The listing builds one solid part. Answer for the finished solid, in the listing's coordinates (mm). A direction names the side the tool comes from. Give positions to 0.01 mm unless a question says otherwise; leave off trailing zeros. Loops run counter-clockwise (first coordinate to the right, second up) from the corner with the lowest first, then second, coordinate; pieces in that order, holes last. Notation, with made-up numbers: M -35.75,-4.5 L -14.75,-4.5 A17 cw -14.75,11.5 Z; hole C 87,39.5 d8. An arc over 180 degrees is marked long. Return JSON: item names as keys, results as strings.
from build123d import *

# Parameters (mm, degrees)
F0_R     = 6.25
F0_R_2   = 2.5
F1_DEPTH = 14
F2_W     = 3.733449
F2_H     = 7
F4_R     = 1.75
F5_DEPTH = 25


with BuildPart() as f1:
    # F0 (on Top) → F1 (new body)
    with BuildSketch(Plane.XY):
        Circle(F0_R)
        Circle(F0_R_2, mode=Mode.SUBTRACT)
    extrude(amount=F1_DEPTH)

    # F2 (on Front) → F3 (revolve, cut)
    with BuildSketch(Plane.XZ):
        with Locations((-6.866725, 8.717095)):
            Rectangle(F2_W, F2_H)
    revolve(axis=Axis((0, 0, 7.230911), (0, 0, -1)), mode=Mode.SUBTRACT)

    # F4 (on Front) → F5 (cut)
    with BuildSketch(Plane.XZ):
        with Locations((0, 2.5)):
            Circle(F4_R)
    extrude(amount=-F5_DEPTH, mode=Mode.SUBTRACT)


solid = f1.part
(1) The part is cut by section A-A (y = 0). Determine the outline of the cut face in (x, z).
Values follow:
{"outline": "M -6.25,0 L -2.5,0 L -2.5,14 L -6.25,14 L -6.25,12.22 L -5,12.22 L -5,5.22 L -6.25,5.22 Z; M 2.5,0 L 6.25,0 L 6.25,5.22 L 5,5.22 L 5,12.22 L 6.25,12.22 L 6.25,14 L 2.5,14 Z"}
(2) Determine the mould class of faces 4 (the cylindrical face through (5.96, 1.88, 13.1)), 5 (the cylindrical face through (-0.54, -2.44, 6.9)), 6 (the flat face through (-2, 5, 12.217)) for opening direction Y: released by +Y, released by -Y, zero draft, split by the parting line, or undercut.
Values follow:
{"face 4": "split by the parting line", "face 5": "undercut", "face 6": "zero draft"}
(3) The part is cut by section D-D (z = 2.5). Determine the outline of the cut face in (x, y).
Values follow:
{"outline": "M -1.75,1.79 L -1.75,6 A6.25 ccw long 1.75,6 L 1.75,1.79 A2.5 cw long Z"}
(4) The part is cut by section C-C (x = 3.5). Determine the outline of the cut face in (y, z), and give its area (3 significant figures).
Values follow:
{"outline": "M -5.18,0 L 5.18,0 L 5.18,5.22 L 3.57,5.22 L 3.57,12.22 L 5.18,12.22 L 5.18,14 L -5.18,14 L -5.18,12.22 L -3.57,12.22 L -3.57,5.22 L -5.18,5.22 Z", "area": "122 mm²"}
(5) Straight lines are drawn through the part: line 1 along Y through (x, z) = (0, 6); line 2 along Z through (x, y) = (-1.5, 5.5); line 3 along Z through (x, y) = (0, 3.7). For each, find the intervals that lie inside material, in ascending order.
Values follow:
{"line 1": "-5 to -2.5, 2.5 to 5", "line 2": "0 to 1.6, 3.4 to 5.22, 12.22 to 14", "line 3": "0 to 0.75, 4.25 to 14"}
(6) The part is cut by section B-B (x = -1.5). Determine the outline of the cut face in (y, z), and give its area (3 significant figures).
Values follow:
{"outline": "M -6.07,0 L -2,0 L -2,14 L -6.07,14 L -6.07,12.22 L -4.77,12.22 L -4.77,5.22 L -6.07,5.22 Z; M 2,0 L 6.07,0 L 6.07,1.6 L 2,1.6 Z; M 2,3.4 L 6.07,3.4 L 6.07,5.22 L 4.77,5.22 L 4.77,12.22 L 6.07,12.22 L 6.07,14 L 2,14 Z", "area": "88.4 mm²"}
(7) Given pin 1 (1 mm diameter, centred on x = 1, z = 9, fed in from -Y); pin 2 (6 mm diameter, centred on y = -5, z = 3, fed in from -X); pin 3 (2 mm diameter, centred on y = 0.5, z = 6.5, fed in from +X); pin 4 (1.5 mm diameter, centred on x = 4.5, y = -2.5, fed in from -Z), each flat-ended and moving along its own axis, determine where each tip first touches the part or whether it passes through.
Values follow:
{"pin 1": "y = -4.97", "pin 2": "x = -5.92", "pin 3": "x = 5", "pin 4": "z = 0"}
(8) A tool of negligible diameter and unlimited length cuts with its end or side. For faces 1 (the cylindrical face through (-4.77, 1.5, 8.77)), 2 (the flat face through (0, -3, 0)), 3 (the cylindrical face through (1.617, 3.99, 1.83)), from which of +Z, -Z, +X, -X, +Y, -Y can it reach the whole face along a straight path? Write none if from no direction.
Values follow:
{"face 1": "none", "face 2": "-Z, +X, -X, +Y, -Y", "face 3": "+Y"}
